Here's the drawing with two shaded views (mm, measured from the low corner). I have some questions. A direction names the side the tool comes from. Round coordinates to 2 decimals unless told otherwise and drop trailing zeros. Loops run counter-clockwise (first coordinate to the right, second up) from the corner with the lowest first, then second, coordinate; pieces in that order, holes last. Notation, with made-up numbers: M 18.25,67.25 L 29.25,67.25 A18 cw 29.25,71.25 Z; hole C 60,80.25 d6. An arc over 180 degrees is marked long. Write each question's results on one line, items separated by ' | '. Start each with the question number.
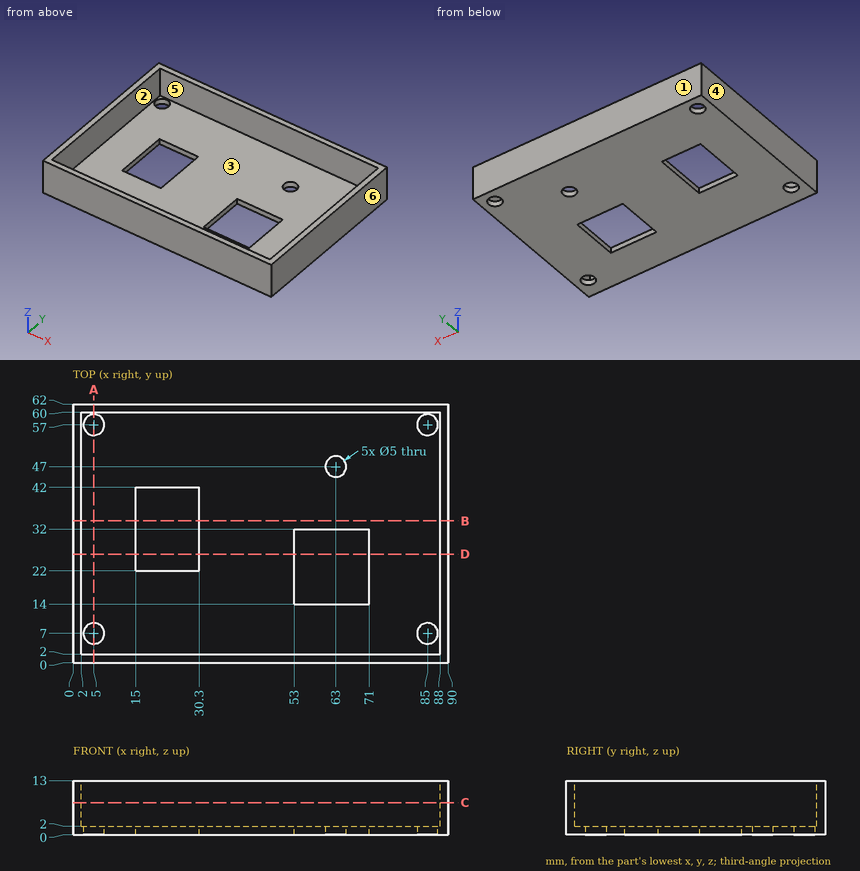
Item 1: If we section it at B-B on y = 34: Please give me the cut outline in (x, z), and give its area (3 significant figures).
Item 2: If we section it at A-A on x = 5: Please give me the cut outline in (y, z).
Item 3: Which directions (+Z, -Z, +X, -X, +Y, -Y) give clear straight access to the entire face, cutting with the end or side of a thin tool? Please do the marked faces 1 and 2.
Item 4: If we section it at C-C on z = 7.75: Please give me the cut outline in (x, y).
Item 5: If we section it at D-D on y = 26: Please give me the cut outline in (x, z), and give its area (3 significant figures).
Item 6: I'm going to push a flat-ended pin straight in: pin 1 (5 mm diameter, centred on x = 79.5, y = 28.5, fed in from +Z). Where does the tip first touch, or does it pass through?
Item 7: I need wall thicknesses on L1, parallel to Y at x = 5, z = 1.4; L2, parallel to Y at x = 63, z = 1.4; L3, parallel to Y at x = 66.5, z = 11. Which ranges of each line are inside material? Lowest first, please.
Item 8: If we mould it in two halves opening along X, with no side actions, what happens to the marked faces 3, 4, 5 and 6? For each: released by +X, released by -X, zero draft, split by the parting line, or undercut.
Numbers:
1) outline: M 0,0 L 15,0 L 15,2 L 2,2 L 2,13 L 0,13 Z; M 30.3,0 L 90,0 L 90,13 L 88,13 L 88,2 L 30.3,2 Z | area: 193 mm²
2) outline: M 0,0 L 4.5,0 L 4.5,2 L 2,2 L 2,13 L 0,13 Z; M 9.5,0 L 54.5,0 L 54.5,2 L 9.5,2 Z; M 59.5,0 L 62,0 L 62,13 L 60,13 L 60,2 L 59.5,2 Z
3) face 1: +Z, -Z, +X, -X, +Y | face 2: +Z
4) outline: M 0,0 L 90,0 L 90,62 L 0,62 Z; hole M 2,2 L 88,2 L 88,60 L 2,60 Z
5) outline: M 0,0 L 15,0 L 15,2 L 2,2 L 2,13 L 0,13 Z; M 30.3,0 L 53,0 L 53,2 L 30.3,2 Z; M 71,0 L 90,0 L 90,13 L 88,13 L 88,2 L 71,2 Z | area: 157 mm²
6) pin 1: z = 2
7) L1: 0 to 4.5, 9.5 to 54.5, 59.5 to 62 | L2: 0 to 14, 32 to 44.5, 49.5 to 62 | L3: 0 to 2, 60 to 62
8) face 3: undercut | face 4: released by -X | face 5: undercut | face 6: released by +X
